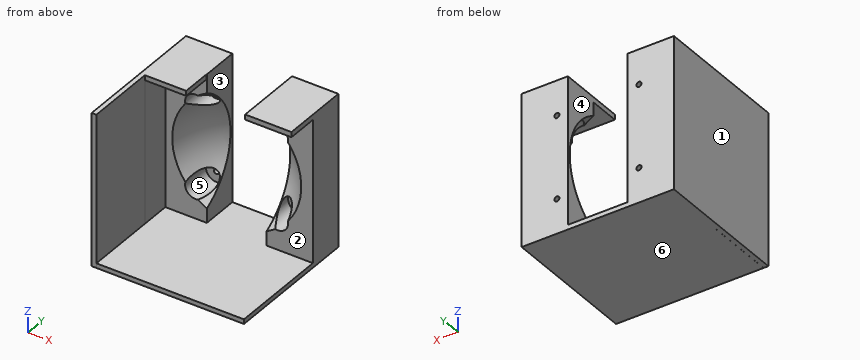
from build123d import *
from build123d.topology import SkipClean

# Parameters (mm, degrees)
SKETCH1_W                   = 102
SKETCH1_H                   = 102
BOSS_EXTRUDE1_DEPTH         = 50
CUT_EXTRUDE_THIN1_OUTLINE_W = 40
CUT_EXTRUDE_THIN1_OUTLINE_H = 95.773670058
CUT_EXTRUDE_THIN1_DEPTH     = 50
SKETCH4_W                   = 40
SKETCH4_H                   = 6.202657501
CUT_EXTRUDE3_DEPTH          = 54
SKETCH5_W                   = 33.817621941
SKETCH5_H                   = 102.594578927
CUT_EXTRUDE4_DEPTH          = 20
SKETCH6_W                   = 27.820383201
SKETCH6_H                   = 98.886835029
CUT_EXTRUDE5_DEPTH          = 20
SKETCH7_W                   = 30.8
SKETCH7_H                   = 3.364819678
BOSS_EXTRUDE2_DEPTH         = 21
SKETCH9_W                   = 31
SKETCH9_H                   = 3.479961613
BOSS_EXTRUDE4_DEPTH         = 21
SKETCH10_W                  = 3.15002448
SKETCH10_H                  = 102
BOSS_EXTRUDE5_DEPTH         = 47.625
SKETCH11_W                  = 98.820383201
SKETCH11_H                  = 3.113164971
BOSS_EXTRUDE6_DEPTH         = 47.625
SKETCH14_W                  = 102
SKETCH14_H                  = 5
CUT_EXTRUDE7_DEPTH          = 105
SKETCH17_R                  = 7
CUT_EXTRUDE12_DEPTH         = 20.5
M3_CLEARANCE_HOLE1_D        = 3.4


# Read off the part's stored shape, not the designer's step: Cut-Extrude-Thin1
with BuildPart() as part:
    # Sketch1 → Boss-Extrude1 (new body)
    with BuildSketch(Plane(origin=(0, 0, 0), x_dir=(1, 0, 0), z_dir=(0, 1, 0))):
        with Locations((-66.567363259, 25.977216604)):
            Rectangle(SKETCH1_W, SKETCH1_H)
    extrude(amount=BOSS_EXTRUDE1_DEPTH)

    # Sketch2 → Cut-Revolve1 (revolve, cut)
    with SkipClean():  # the faces are left unmerged after this step: merging them gives an invalid solid
        with BuildSketch(Plane(origin=(0, 0, 0), x_dir=(1, 0, 0), z_dir=(0, 1, 0))):
            with BuildLine():
                ThreePointArc((-66.567363259, 73.602216604), (-114.192363259, 25.977216604), (-66.567363259, -21.647783396))
                Line((-66.567363259, -21.647783396), (-66.567363259, 73.602216604))
            make_face()
            with BuildLine():
                Line((-66.567363259, 73.602216604), (-66.567363259, -21.647783396))
                ThreePointArc((-66.567363259, -21.647783396), (-32.891402805, -7.69874385), (-18.942363259, 25.977216604))
                ThreePointArc((-18.942363259, 25.977216604), (-32.891402805, 59.653177058), (-66.567363259, 73.602216604))
            make_face()
        revolve(axis=Axis((-66.567363259, 0, 21.647783396), (0, 0, -1)), mode=Mode.SUBTRACT)
    add(part.part.scale(1), mode=Mode.REPLACE)  # the faces are merged on a copy

    # Cut-Extrude-Thin1 outline → Cut-Extrude-Thin1 (cut)
    with BuildSketch(Plane(origin=(0, 0, 0), x_dir=(1, 0, 0), z_dir=(0, 1, 0))):
        with Locations((-66.567363259, 25.977216604)):
            Rectangle(CUT_EXTRUDE_THIN1_OUTLINE_W, CUT_EXTRUDE_THIN1_OUTLINE_H)
    extrude(amount=CUT_EXTRUDE_THIN1_DEPTH, mode=Mode.SUBTRACT)

    # Sketch4 → Cut-Extrude3 (cut)
    with BuildSketch(Plane(origin=(0, 0, 0), x_dir=(1, 0, 0), z_dir=(0, 1, 0))):
        with Locations((-66.567363259, -25.010947176)):
            Rectangle(SKETCH4_W, SKETCH4_H)
    extrude(amount=CUT_EXTRUDE3_DEPTH, mode=Mode.SUBTRACT)

    # Sketch5 → Cut-Extrude4 (cut)
    with BuildSketch(Plane(origin=(0, 0, 0), x_dir=(1, 0, 0), z_dir=(0, 1, 0))):
        with Locations((-29.658552289, 22.56676217)):
            Rectangle(SKETCH5_W, SKETCH5_H)
    extrude(amount=CUT_EXTRUDE4_DEPTH, mode=Mode.SUBTRACT)

    # Sketch6 → Cut-Extrude5 (cut)
    with BuildSketch(Plane(origin=(0, 0, 0), x_dir=(-1, 0, 0), z_dir=(0, -1, 0))):
        with Locations((100.47755486, 24.420634119)):
            Rectangle(SKETCH6_W, SKETCH6_H)
    extrude(amount=-CUT_EXTRUDE5_DEPTH, mode=Mode.SUBTRACT)

    # Sketch7 → Boss-Extrude2 (add)
    with BuildSketch(Plane(origin=(0, 0, 0), x_dir=(1, 0, 0), z_dir=(0, 1, 0))):
        with Locations((-102.167363259, -23.340373557)):
            Rectangle(SKETCH7_W, SKETCH7_H)
    extrude(amount=BOSS_EXTRUDE2_DEPTH)

    # Sketch9 → Boss-Extrude4 (add)
    with BuildSketch(Plane.XZ.offset(-20)):
        with Locations((-31.067363259, 23.28280259)):
            Rectangle(SKETCH9_W, SKETCH9_H)
    extrude(amount=BOSS_EXTRUDE4_DEPTH)

    # Sketch10 → Boss-Extrude5 (add)
    with BuildSketch(Plane.XZ):
        with Locations((-115.992351019, -25.977216604)):
            Rectangle(SKETCH10_W, SKETCH10_H)
    extrude(amount=BOSS_EXTRUDE5_DEPTH)

    # Sketch11 → Boss-Extrude6 (add)
    with BuildSketch(Plane.XZ):
        with Locations((-64.97755486, -75.420634119)):
            Rectangle(SKETCH11_W, SKETCH11_H)
    extrude(amount=BOSS_EXTRUDE6_DEPTH)

    # Sketch14 → Cut-Extrude7 (cut)
    with BuildSketch(Plane(origin=(-15.567363259, 0, 0), x_dir=(0, 0, -1), z_dir=(1, 0, 0))):
        with Locations((25.977216604, 47.5)):
            Rectangle(SKETCH14_W, SKETCH14_H)
    extrude(amount=-CUT_EXTRUDE7_DEPTH, mode=Mode.SUBTRACT)

    # Sketch17 → Cut-Extrude12 (cut)
    with BuildSketch(Plane.XZ.offset(-20)):
        with Locations(Location((-94.167363259, 1.657963718, 0), (0, 0, 270))):
            Circle(SKETCH17_R)
        with Locations(Location((-94.167363259, -53.864051633, 0), (0, 0, 284.685382437))):
            Circle(SKETCH17_R)
        with Locations(Location((-39.167363259, 1.657963718, 0), (0, 0, 349.246729183))):
            Circle(SKETCH17_R)
        with Locations(Location((-39.167363259, -53.864051633, 0), (0, 0, 270))):
            Circle(SKETCH17_R)
    extrude(amount=-CUT_EXTRUDE12_DEPTH, mode=Mode.SUBTRACT)

    # M3 Clearance Hole1 (through all)
    with Locations(Plane(origin=(0, 40.5, 0), x_dir=(-1, 0, 0), z_dir=(0, -1, 0))):
        with Locations((94.167363259, -1.657963718), (39.167363259, -1.657963718), (39.167363259, 53.864051633), (94.167363259, 53.864051633)):
            Hole(M3_CLEARANCE_HOLE1_D / 2)


solid = part.part
Source: CAD feature listing. Evaluate the final solid. Frame: model axes, mm. Face numbers are marked on the shaded views. A direction names the side the tool comes from. Coordinates: 2 decimals unless noted, no trailing zeros. Write each loop counter-clockwise with the first axis right and the second up, starting at its lowest first coordinate (ties: lowest second). Pieces come first, ordered by that corner, then holes. Notation, with made-up numbers: M -1,74 L 10,74 A21 ccw 10,104 Z; hole C 28,-29.5 d2. An arc over 180 degrees is marked long. Use a Markdown table: item, result.
1) Mould query, pull axis Z, two halves, no side actions, for the marked faces 4, 5 and 6. Classes: pulls with the +Z half, pulls with the -Z half, needs draft (parallel to the pull), parting line crosses it, or undercut.
Conclusion:
| item | result |
|---|---|
| face 4 | needs draft |
| face 5 | undercut |
| face 6 | pulls with the -Z half |
2) Section B-B, the plane z = 14. Output: boundary loops of the cut face in (x, y) (3 decimals), then the cut area to 3 significant figures.
Conclusion:
| item | result |
|---|---|
| outline | M -117.567,-47.625 L -114.417,-47.625 L -114.417,0 L -114.388,0 L -114.388,20 L -86.567,20 L -86.567,45 L -117.567,45 Z; M -46.567,20 L -15.567,20 L -15.567,45 L -46.567,45 Z |
| area | 1,760 mm^2 |
3) Section C-C, the plane x = -105. Output: boundary loops of the cut face in (y, z) (3 decimals).
Conclusion:
| item | result |
|---|---|
| outline | M -47.625,-76.977 L 45,-76.977 L 45,25.023 L 0,25.023 L 0,21.658 L 20,21.658 L 20,-6.202 A28.126 cw 20,-45.753 L 20,-73.864 L -47.625,-73.864 Z |
4) First-contact query: pin 1 Ø14 at (x, z) = (-96.5, -2.5) entering from -Y; pin 2 Ø4 at (x, z) = (-97.5, -56.5) entering from -Y; pin 3 Ø1.5 at (x, y) = (-79.5, -4) entering from +Z. Flat tips, straight axial feed; report the tip coordinate or a pass-through.
Conclusion:
| item | result |
|---|---|
| pin 1 | stops at y = 20 |
| pin 2 | stops at y = 40.5 |
| pin 3 | stops at z = -73.86 |
5) Reachability of the marked faces 1, 2 and 3 from +Z, -Z, +X, -X, +Y, -Y: full face, straight path, thin tool, end or side. Return the list, or none.
Conclusion:
| item | result |
|---|---|
| face 1 | +Z, -Z, -X, +Y, -Y |
| face 2 | +X, -Y |
| face 3 | +Z, +Y, -Y |
6) Ray query, L1, parallel to X at y = 35, z = 9; L2, parallel to Z at x = -82, y = 37; L3, parallel to X at y = 39, z = 0. Return the intervals inside material, ascending.
Conclusion:
| item | result |
|---|---|
| L1 | x = -117.57 to -86.57, -46.57 to -15.57 |
| L2 | z = -76.98 to -73.86 |
| L3 | x = -117.57 to -100.97, -87.37 to -86.57, -46.57 to -45.97, -32.37 to -15.57 |
7) Section D-D, the plane y = 27. Output: boundary loops of the cut face in (x, z), then the cut area to 3 significant figures.
Conclusion:
| item | result |
|---|---|
| outline | M -117.57,-76.98 L -15.57,-76.98 L -15.57,25.02 L -46.57,25.02 L -46.57,7.77 A39.23 cw -44.35,6.36 A7 cw long -34.42,-3.49 A39.23 cw -34.53,-48.62 A7 cw long -44.49,-58.41 A39.23 cw -46.57,-59.73 L -46.57,-73.86 L -86.57,-73.86 L -86.57,-59.73 A39.23 cw -88.77,-58.32 A7 cw long -98.68,-48.51 A39.23 cw -98.79,-3.6 A7 cw long -88.91,6.27 A39.23 cw -86.57,7.77 L -86.57,25.02 L -117.57,25.02 Z |
| area | 4,300 mm^2 |
8) Section A-A, the plane y = -17. Output: boundary loops of the cut face in (x, z).
Conclusion:
| item | result |
|---|---|
| outline | M -117.57,-76.98 L -114.42,-76.98 L -114.42,25.02 L -117.57,25.02 Z; M -114.39,-76.98 L -15.57,-76.98 L -15.57,-73.86 L -114.39,-73.86 Z |
